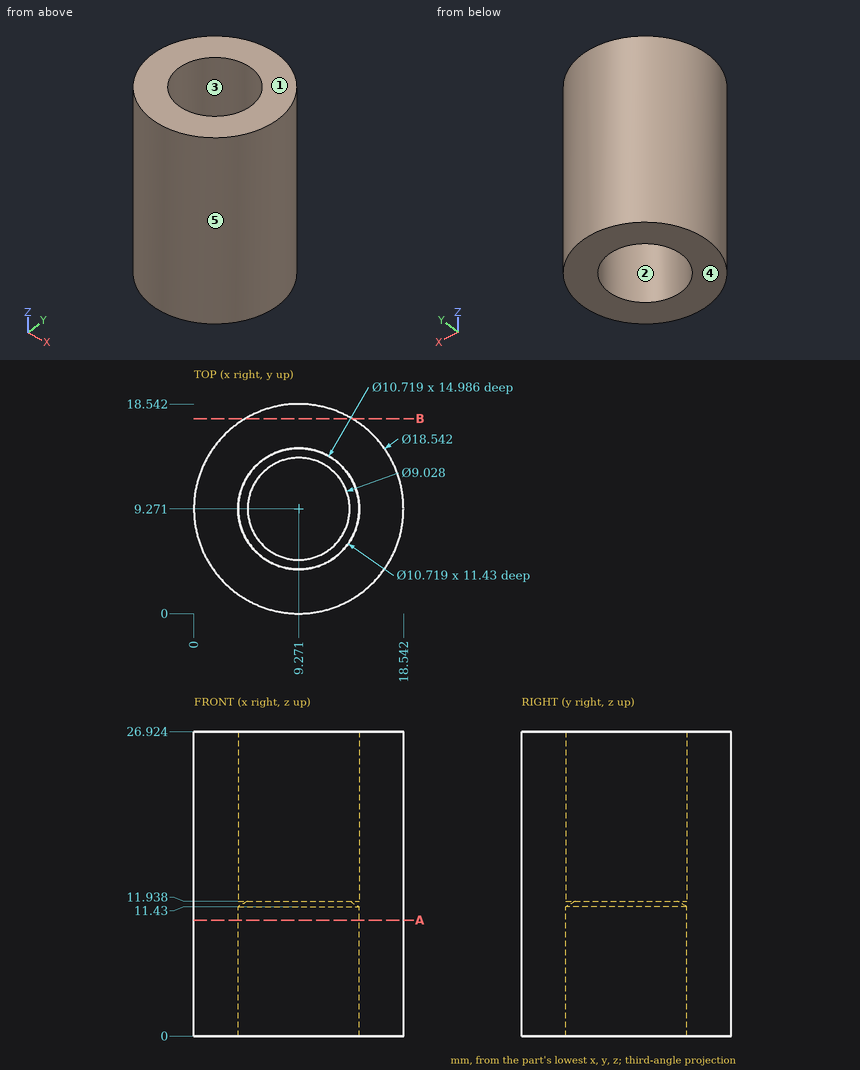
Check sheet for the drawn part. Datum: minimum x, y, z corner. Units: mm. A direction names the side the tool comes from. Round coordinates to 2 decimals unless told otherwise and drop trailing zeros. Order: outer loops, then holes, each group sorted by start corner. A loop starts at its lowest first (then second) coordinate and runs counter-clockwise, first axis right, second up. Notation, with made-up numbers: (27.25, -29.75) -> (38.25, -29.75) arc R35 cw to (38.25, 8.25) -> close; hole circle Ø11 at (66.5, -29.75). An arc over 180 degrees is marked (long way). Return JSON: item names as keys, results as strings. Group by question number.
Q1. Gauge pin test, flat ends, axial feed: pin 1 (2 mm diameter, centred on y = 14.5, z = 4, fed in from +X); pin 2 (5 mm diameter, centred on x = 13, z = 22, fed in from +Y); pin 3 (4 mm diameter, centred on x = 14.5, z = 4, fed in from -Y); pin 4 (2 mm diameter, centred on y = 10, z = 19.5, fed in from +X). Record the tip position at first contact, or that the pin passes through.
Q2. Material ranges on probe 1 along Y at (x, z) = (9.5, 8); probe 2 along X at (y, z) = (5, 21.25); probe 3 along Y at (x, z) = (9.5, 11.75), recorded low to high. Write a range as from..to.
Q3. Release check for a two-part mould opening along X. For the marked faces 3, 4 and 5 record: released by +X, released by -X, zero draft, split by the parting line, or undercut.
Q4. Tool access check on the marked faces 1 and 2. Record the directions out of +Z, -Z, +X, -X, +Y, -Y that give a thin tool (end or side, any length) a straight path to the whole face; none if there is none.
Q5. Section check B-B, the plane y = 17.25. Record the boundary of the cut face in (x, z), plus the area to 3 significant figures.
Q6. Section check A-A, the plane z = 10.25. Record the boundary of the cut face in (x, y), plus the area to 3 significant figures.
Numbers:
{
 "1": {"pin 1": "x = 17.52", "pin 2": "y = 18.46", "pin 3": "y = 0.58", "pin 4": "x = 18.54"},
 "2": {"probe 1": "0..3.92, 14.63..18.54", "probe 2": "1.04..6.03, 12.51..17.5", "probe 3": "0..4.45, 14.09..18.54"},
 "3": {"face 3": "undercut", "face 4": "zero draft", "face 5": "split by the parting line"},
 "4": {"face 1": "+Z, +X, -X, +Y, -Y", "face 2": "-Z"},
 "5": {"outline": "(4.55, 0) -> (13.99, 0) -> (13.99, 26.92) -> (4.55, 26.92) -> close", "area": "254 mm^2"},
 "6": {"outline": "circle Ø18.54 at (9.27, 9.27); hole circle Ø10.72 at (9.27, 9.27)", "area": "180 mm^2"}
}
